from build123d import *

# Parameters (mm, degrees)
SKETCH1_R           = 16.5
SKETCH1_R_2         = 15
BOSS_EXTRUDE1_DEPTH = 44
SKETCH3_W           = 13
SKETCH3_H           = 3.5
CUT_EXTRUDE1_DEPTH  = 44


with BuildPart() as part:
    # Sketch1 → Boss-Extrude1 (new body)
    with BuildSketch(Plane(origin=(0, 0, 0), x_dir=(1, 0, 0), z_dir=(0, 1, 0))):
        with Locations(Location((0, 0, 0), (0, 0, 270))):
            Circle(SKETCH1_R)
        with Locations(Location((0, 0, 0), (0, 0, 270))):
            Circle(SKETCH1_R_2, mode=Mode.SUBTRACT)
    extrude(amount=BOSS_EXTRUDE1_DEPTH)

    # Sketch3 → Cut-Extrude1 (cut)
    with BuildSketch(Plane.XY):
        with Locations((0, 1.75)):
            Rectangle(SKETCH3_W, SKETCH3_H)
        with Locations((0, 42.25)):
            Rectangle(SKETCH3_W, SKETCH3_H)
    extrude(amount=-CUT_EXTRUDE1_DEPTH, mode=Mode.SUBTRACT)


solid = part.part
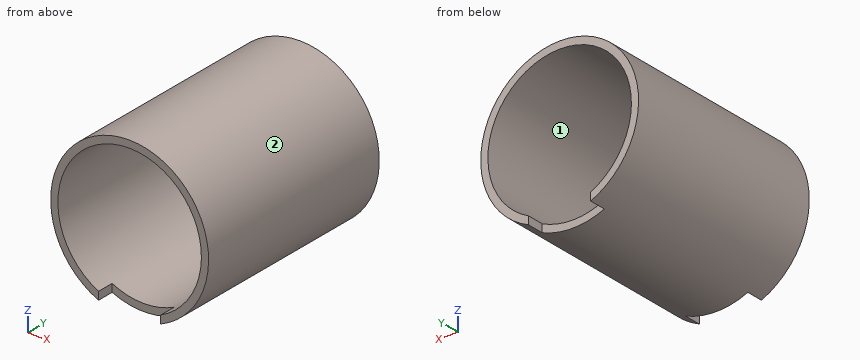
Geometry: final body of the model. Coordinates: model frame, mm. Face numbers are marked on the shaded views. Round coordinates to 2 decimals unless told otherwise and drop trailing zeros. Loops run counter-clockwise (first coordinate to the right, second up) from the corner with the lowest first, then second, coordinate; pieces in that order, holes last.
Q1. Section B-B on z = 0. Return loops of the section in (x, y), plus the area to 3 significant figures.
Q2. Pull-direction query (X, two-part tool) for the marked faces 1 and 2; classes: released by +X, released by -X, zero draft, split by the parting line, or undercut.
Q3. Section A-A on x = 0. Return loops of the section in (y, z).
Q4. Material intervals for L1, parallel to X at y = 24.5, z = 0; L2, parallel to Z at x = 7, y = 25.5; L3, parallel to X at y = 14, z = 12, sorted ascending.
Q5. Pin query (flat end, axial travel): P1, Ø4, axis at y = 28, z = -10.5, coming from the -X side; P2, Ø2.5, axis at x = -1.5, z = -15.5, coming from the -Y side; P3, Ø1.3, axis at y = 2.5, z = -14.5, coming from the +X side; P4, Ø4, axis at x = -0.5, y = 14, coming from the -Z side. Return the tip coordinate at first contact, or that it passes through.
Q6. Section C-C on y = 35. Return loops of the section in (x, z).
Evaluation:
1. outline: (-16.5, 0) - (-15, 0) - (-15, 44) - (-16.5, 44) - close; (15, 0) - (16.5, 0) - (16.5, 44) - (15, 44) - close
1. area: 132 mm2
2. face 1: undercut
2. face 2: split by the parting line
3. outline: (0, 15) - (44, 15) - (44, 16.5) - (0, 16.5) - close; (3.5, -16.5) - (40.5, -16.5) - (40.5, -15) - (3.5, -15) - close
4. L1: x = -16.5 to -15, 15 to 16.5
4. L2: z = -14.94 to -13.27, 13.27 to 14.94
4. L3: x = -11.32 to -9, 9 to 11.32
5. P1: stops at x = -14.14
5. P2: stops at y = 3.5
5. P3: stops at x = 8.97
5. P4: stops at z = -16.5
6. outline: circle Ø33 at (0, 0); hole circle Ø30 at (0, 0)
